```python
from build123d import *

# Parameters (mm, degrees)
CROQUIS1_W              = 38
CROQUIS1_H              = 9
SALIENTE_EXTRUIR1_DEPTH = 2
CORTAR_EXTRUIR1_REACH   = 21.628
CROQUIS2_R              = 1.5


with BuildPart() as part:
    # Croquis1 → Saliente-Extruir1 (new body)
    with BuildSketch(Plane(origin=(0, 0, 0), x_dir=(1, 0, 0), z_dir=(0, 1, 0))):
        Rectangle(CROQUIS1_W, CROQUIS1_H)
    extrude(amount=SALIENTE_EXTRUIR1_DEPTH)

    # Croquis2 → Cortar-Extruir1 (cut, up to next)
    with BuildSketch(Plane(origin=(0, 2, 0), x_dir=(1, 0, 0), z_dir=(0, 1, 0)), mode=Mode.PRIVATE) as cortar_extruir1_sk1:
        with Locations(Location((-15.5, 0, 0), (0, 0, 270))):
            Circle(CROQUIS2_R)
    cortar_extruir1_tool1 = extrude(cortar_extruir1_sk1.sketch, amount=-CORTAR_EXTRUIR1_REACH, mode=Mode.PRIVATE) & part.part
    # Croquis2 → Cortar-Extruir1 (cut, up to next)
    with BuildSketch(Plane(origin=(0, 2, 0), x_dir=(1, 0, 0), z_dir=(0, 1, 0)), mode=Mode.PRIVATE) as cortar_extruir1_sk2:
        with Locations(Location((15.5, 0, 0), (0, 0, 90))):
            Circle(CROQUIS2_R)
    cortar_extruir1_tool2 = extrude(cortar_extruir1_sk2.sketch, amount=-CORTAR_EXTRUIR1_REACH, mode=Mode.PRIVATE) & part.part
    add(cortar_extruir1_tool1.solids().sort_by_distance((-15.5, 2, 0))[0], mode=Mode.SUBTRACT)
    add(cortar_extruir1_tool2.solids().sort_by_distance((15.5, 2, 0))[0], mode=Mode.SUBTRACT)


solid = part.part
```
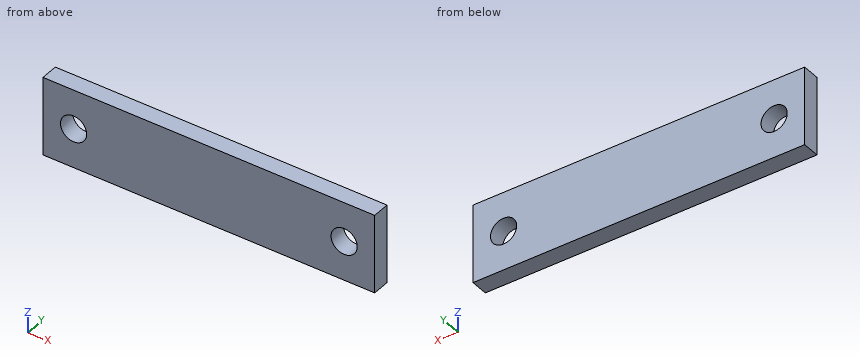
Geometry: final body of the model. Coordinates: model frame, mm. Give positions to 0.01 mm unless a question says otherwise; leave off trailing zeros. Order: outer loops, then holes, each group sorted by start corner. A loop starts at its lowest first (then second) coordinate and runs counter-clockwise, first axis right, second up. Notation, with made-up numbers: (43, 86.25) -> (94, 86.25) arc R19 ccw to (94, 104.25) -> close; hole circle Ø8 at (-19.75, 51.25). An arc over 180 degrees is marked (long way). Write each question's results on one line, items separated by ' | '. Start each with the question number.
1) Section C-C (y = 0.35). Return loops of the section in (x, z).
2) First-contact query: pin 1 (2.5 mm diameter, centred on x = 15.5, z = 0, fed in from -Y). Flat tip, straight axial feed; report the tip coordinate or a pass-through.
3) Section B-B (x = 15.5). Return loops of the section in (y, z).
4) Section A-A (z = 0). Return loops of the section in (x, y), then the cut area to 3 significant figures.
5) Line query: line 1 (X direction, y = 0.5, z = 0); line 2 (Z direction, x = 15.5, y = 1.4); line 3 (X direction, y = 1, z = 0.5). Output: solid intervals per line, ascending. Write a range as from..to.
Calculated:
1) outline: (-19, -4.5) -> (19, -4.5) -> (19, 4.5) -> (-19, 4.5) -> close; hole circle Ø3 at (-15.5, 0); hole circle Ø3 at (15.5, 0)
2) pin 1: through
3) outline: (0, -4.5) -> (2, -4.5) -> (2, -1.5) -> (0, -1.5) -> close; (0, 1.5) -> (2, 1.5) -> (2, 4.5) -> (0, 4.5) -> close
4) outline: (-19, 0) -> (-17, 0) -> (-17, 2) -> (-19, 2) -> close; (-14, 0) -> (14, 0) -> (14, 2) -> (-14, 2) -> close; (17, 0) -> (19, 0) -> (19, 2) -> (17, 2) -> close | area: 64.0 mm2
5) line 1: -19..-17, -14..14, 17..19 | line 2: -4.5..-1.5, 1.5..4.5 | line 3: -19..-16.91, -14.09..14.09, 16.91..19
